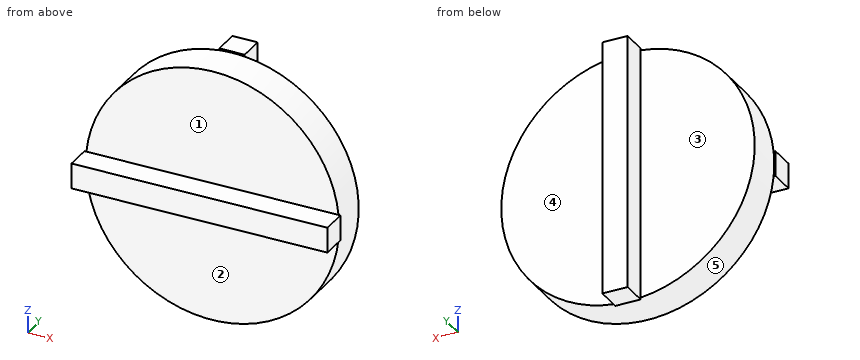
```python
from build123d import *

# Parameters (mm, degrees)
SKETCH1_R           = 50
BOSS_EXTRUDE1_DEPTH = 15
SKETCH2_W           = 10
SKETCH2_H           = 101
BOSS_EXTRUDE2_DEPTH = 10
SKETCH3_W           = 101
SKETCH3_H           = 10
BOSS_EXTRUDE3_DEPTH = 10


with BuildPart() as part:
    # Sketch1 → Boss-Extrude1 (new body)
    with BuildSketch(Plane(origin=(0, 0, 0), x_dir=(1, 0, 0), z_dir=(0, 1, 0))):
        with Locations(Location((0, 0, 0), (0, 0, 270))):
            Circle(SKETCH1_R)
    extrude(amount=BOSS_EXTRUDE1_DEPTH)

    # Sketch2 → Boss-Extrude2 (add)
    with BuildSketch(Plane(origin=(0, 15, 0), x_dir=(1, 0, 0), z_dir=(0, 1, 0))):
        Rectangle(SKETCH2_W, SKETCH2_H)
    extrude(amount=BOSS_EXTRUDE2_DEPTH)

    # Sketch3 → Boss-Extrude3 (add)
    with BuildSketch(Plane.XZ):
        Rectangle(SKETCH3_W, SKETCH3_H)
    extrude(amount=BOSS_EXTRUDE3_DEPTH)


solid = part.part
```
The listing builds one solid part. Answer for the finished solid, in the listing's coordinates (mm). Face numbers are marked on the shaded views. A direction names the side the tool comes from. Round coordinates to 2 decimals unless told otherwise and drop trailing zeros. Loops run counter-clockwise (first coordinate to the right, second up) from the corner with the lowest first, then second, coordinate; pieces in that order, holes last.
1) A cutting plane is placed at B-B on z = 0. Determine the outline of the cut face in (x, y).
Outcome:
outline: (-50.5, -10) - (50.5, -10) - (50.5, 0) - (50, 0) - (50, 15) - (5, 15) - (5, 25) - (-5, 25) - (-5, 15) - (-50, 15) - (-50, 0) - (-50.5, 0) - close
2) Consider line 1 (Y direction, x = -11, z = 13); line 2 (Z direction, x = 24, y = -2); line 3 (Y direction, x = -0.5, z = -11.5). Determine where each line is inside the solid, lowest interval first.
Outcome:
line 1: y = 0 to 15
line 2: z = -5 to 5
line 3: y = 0 to 25
3) For the marked faces 1, 2 and 3, determine the directions among +Z, -Z, +X, -X, +Y, -Y from which every point of the face is accessible in a straight line to the end or side of a thin tool.
Outcome:
face 1: +Z, +X, -X, -Y
face 2: -Z, +X, -X, -Y
face 3: +Z, -Z, -X, +Y
4) A cutting plane is placed at D-D on x = 40. Determine the outline of the cut face in (y, z).
Outcome:
outline: (-10, -5) - (0, -5) - (0, -30) - (15, -30) - (15, 30) - (0, 30) - (0, 5) - (-10, 5) - close
5) Given P1, Ø11, axis at y = 19, z = 7, coming from the +X side; P2, Ø5, axis at y = 5, z = -18, coming from the -X side; P3, Ø22.5, axis at x = -21, z = 21.5, coming from the -Y side, each flat-ended and moving along its own axis, determine where each tip first touches the part or whether it passes through.
Outcome:
P1: stops at x = 49.9
P2: stops at x = -47.54
P3: stops at y = 0
6) A cutting plane is placed at C-C on y = 3. Determine the outline of the cut face in (x, z), plus the area to 3 significant figures.
Outcome:
outline: circle Ø100 at (0, 0)
area: 7,850 mm2
7) For a pull along Z with two mould halves and no side action, classify the marked faces 4 and 5 as released by +Z, released by -Z, zero draft, split by the parting line, or undercut.
Outcome:
face 4: zero draft
face 5: split by the parting line
8) A cutting plane is placed at A-A on x = 0. Determine the outline of the cut face in (y, z).
Outcome:
outline: (-10, -5) - (0, -5) - (0, -50) - (15, -50) - (15, -50.5) - (25, -50.5) - (25, 50.5) - (15, 50.5) - (15, 50) - (0, 50) - (0, 5) - (-10, 5) - close
